Work out the finished part from the listing and answer in its coordinate system (mm). Face numbers are marked on the shaded views. A direction names the side the tool comes from. Coordinates: 2 decimals unless noted, no trailing zeros. Write each loop counter-clockwise with the first axis right and the second up, starting at its lowest first coordinate (ties: lowest second). Pieces come first, ordered by that corner, then holes. Notation, with made-up numbers: (-5, 49.5) - (17, 49.5) arc R22 cw to (17, 83.5) - close; hole circle Ø4 at (-23.75, 31). An arc over 180 degrees is marked (long way). Use one line per item in the form item = value. Start each with the question number.
Item 1: A cutting plane is placed at D-D (x = 5.75). Write down the section's boundary in (y, z), then the cut area to 3 significant figures.
Item 2: Determine the mould class of the marked faces 1, 2 and 3 for opening direction Y: released by +Y, released by -Y, zero draft, split by the parting line, or undercut.
Item 3: A cutting plane is placed at C-C (z = 7.25). Write down the section's boundary in (x, y).
Item 4: Consider probe 1 along Y at (x, z) = (0, 7.65); probe 2 along Z at (x, y) = (-2.75, 2.25); probe 3 along X at (y, z) = (-3, 7.5). Determine where each line is inside the solid, lowest interval first.
Item 5: Given pin 1 (6.5 mm diameter, centred on x = 0, y = 0, fed in from +Z); pin 2 (5 mm diameter, centred on y = -3, z = 1.5, fed in from +X); pin 3 (1.5 mm diameter, centred on x = -5, z = 7, fed in from -Y), each flat-ended and moving along its own axis, determine where each tip first touches the part or whether it passes through.
Item 6: A cutting plane is placed at A-A (y = 0). Write down the section's boundary in (x, z).
Item 7: For the marked faces 4 and 5, determine the directions among +Z, -Z, +X, -X, +Y, -Y from which every point of the face is accessible in a straight line to the end or side of a thin tool.
Autodesk Inventor part; units mm, degrees
ref_plane "YZ Plane" through (0, 0, 0) normal (1, 0, 0) x (0, 1, 0)
ref_plane "XZ Plane" through (0, 0, 0) normal (0, 1, 0) x (-1, 0, 0)
ref_plane "XY Plane" through (0, 0, 0) normal (0, 0, 1) x (1, 0, 0)
sketch "Sketch1" plane through (0, 0, 0) normal (0, 0, 1) x (1, 0, 0)
  circle A0 centre (0, 0) radius 7.95
  dimension "d0" = 15.9
extrude "Extrusion1" add sketch "Sketch1" along normal blind 8.95
sketch "Sketch2" plane through (0, 0, 8.95) normal (0, 0, 1) x (1, 0, 0)
  circle A0 centre (0, 0) radius 3.6
  dimension "d3" = 7.2
extrude "Extrusion2" cut sketch "Sketch2" against normal blind 2.6
sketch "Sketch3" plane through (0, 0, 6.35) normal (0, 0, 1) x (1, 0, 0)
  circle A0 centre (0, 0) radius 2.2
  dimension "d6" = 4.4
extrude "Extrusion3" cut sketch "Sketch3" against normal up to next
properties part number "E3Dv6Spacer"
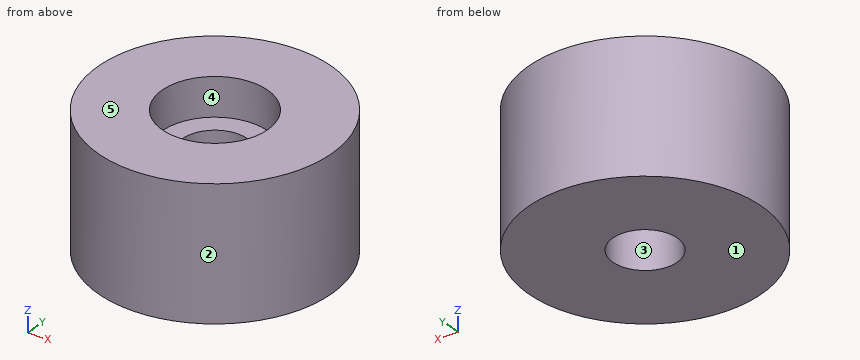
Answer:
q1.outline = (-5.49, 0) - (5.49, 0) - (5.49, 8.95) - (-5.49, 8.95) - close
q1.area = 98.3 mm²
q2.face_1 = zero draft
q2.face_2 = split by the parting line
q2.face_3 = undercut
q3.outline = circle Ø15.9 at (0, 0); hole circle Ø7.2 at (0, 0)
q4.probe_1 = -7.95 to -3.6, 3.6 to 7.95
q4.probe_2 = 0 to 6.35
q4.probe_3 = -7.36 to -1.99, 1.99 to 7.36
q5.pin_1 = 6.35
q5.pin_2 = 7.93
q5.pin_3 = -6.72
q6.outline = (-7.95, 0) - (-2.2, 0) - (-2.2, 6.35) - (-3.6, 6.35) - (-3.6, 8.95) - (-7.95, 8.95) - close; (2.2, 0) - (7.95, 0) - (7.95, 8.95) - (3.6, 8.95) - (3.6, 6.35) - (2.2, 6.35) - close
q7.face_4 = +Z
q7.face_5 = +Z, +X, -X, +Y, -Y
